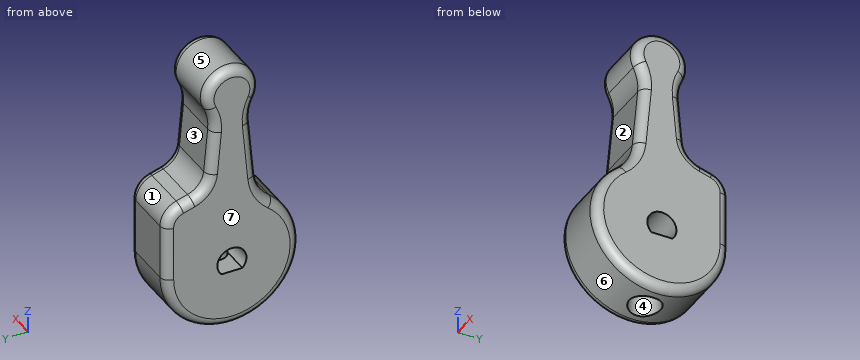
from build123d import *

# Parameters (mm, degrees)
BOSS_EXTRUDE1_DEPTH = 3.5
FILLET1_R           = 5
HOLE1_D             = 2.5
HOLE1_DEPTH         = 8
HOLE1_CBORE_D       = 3.5
HOLE1_CBORE_DEPTH   = 3
BOSS_EXTRUDE2_DEPTH = 7
FILLET3_R           = 2.5
FILLET2_R           = 1


with BuildPart() as part:
    # Sketch1 → Boss-Extrude1 (new, symmetric)
    with BuildSketch(Plane(origin=(0, 0, 0), x_dir=(0, 0, -1), z_dir=(1, 0, 0))):
        with BuildLine():
            Line((-17.763932023, 2), (-6.873863542, 3))
            ThreePointArc((-6.873863542, 3), (7.5, 0), (-6.873863542, -3))
            Line((-6.873863542, -3), (-17.763932023, -2))
            ThreePointArc((-17.763932023, -2), (-23, 0), (-17.763932023, 2))
        make_face()
        with BuildLine():
            Line((1.125, -1.17260394), (1.125, 1.17260394))
            ThreePointArc((1.125, 1.17260394), (-1.625, 0), (1.125, -1.17260394))
        make_face(mode=Mode.SUBTRACT)
    extrude(amount=BOSS_EXTRUDE1_DEPTH, both=True)

    # Fillet1
    fillet1_edges = [part.edges().sort_by_distance(p)[0] for p in [
        (0, 2, 17.763932023),
        (0, 3, 6.873863542),
        (0, -3, 6.873863542),
        (0, -2, 17.763932023),
    ]]
    fillet(fillet1_edges, radius=FILLET1_R)

    # Hole1
    with Locations(Plane(origin=(0, 0, -7.625), x_dir=(1, 0, 0), z_dir=(0, 0, -1))):
        with Locations((0, 0)):
            CounterBoreHole(HOLE1_D / 2, HOLE1_CBORE_D / 2, HOLE1_CBORE_DEPTH, depth=HOLE1_DEPTH)

    # Sketch4 → Boss-Extrude2 (add, through all)
    with BuildSketch(Plane(origin=(3.5, 0, 0), x_dir=(0, 0, -1), z_dir=(1, 0, 0))):
        with BuildLine():
            Line((0, 7.5), (-8, 7.5))
            Line((-8, 7.5), (-9.348908132, 2.772724607))
            ThreePointArc((-9.348908132, 2.772724607), (-7.423390623, 3.356027744), (-5.883671087, 4.651065957))
            ThreePointArc((-5.883671087, 4.651065957), (-3.268562782, 6.750296093), (0, 7.5))
        make_face()
    extrude(amount=-BOSS_EXTRUDE2_DEPTH)

    # Fillet3
    fillet3_edges = [part.edges().sort_by_distance(p)[0] for p in [
        (0, 2.772724607, 9.348908132),
        (0, 7.5, 8),
    ]]
    fillet(fillet3_edges, radius=FILLET3_R)

    # Fillet2
    fillet2_edges = [part.edges().sort_by_distance(p)[0] for p in [
        (-3.5, 0, 23),
        (3.5, 0, 23),
        (-3.5, -3.268562782, -6.750296093),
        (3.5, -3.268562782, -6.750296093),
        (-3.5, -2.469818808, 12.647573032),
        (3.5, -2.469818808, 12.647573032),
        (-3.5, 2.233464618, 17.334759204),
        (3.5, 2.233464618, 17.334759204),
        (-3.5, -3.356027744, 7.423390623),
        (3.5, -3.356027744, 7.423390623),
        (-3.5, -2.233464618, 17.334759204),
        (3.5, -2.233464618, 17.334759204),
        (-3.5, 7.5, 3.056789081),
        (3.5, 7.5, 3.056789081),
        (-3.5, 2.391513819, 13.50031972),
        (3.5, 2.391513819, 13.50031972),
        (3.5, 5.052820312, 8.698292421),
        (-3.5, 5.052820312, 8.698292421),
        (3.5, 6.995615118, 7.619406937),
        (-3.5, 6.995615118, 7.619406937),
        (-3.5, 3.181037085, 9.687418633),
        (3.5, 3.181037085, 9.687418633),
    ]]
    fillet(fillet2_edges, radius=FILLET2_R)


solid = part.part
Design review of the part built by this model. Coordinates are the model's own, in mm. Face numbers are marked on the shaded views. A direction names the side the tool comes from. Give positions to 0.01 mm unless a question says otherwise; leave off trailing zeros. Write each loop counter-clockwise with the first axis right and the second up, starting at its lowest first coordinate (ties: lowest second). Pieces come first, ordered by that corner, then holes. Notation, with made-up numbers: M 36,6.25 L 74,6.25 A25 ccw 74,35.25 Z; hole C 33,-31.75 d2. An arc over 180 degrees is marked long. Answer as a JSON object with one key per item and string values. Group by question number.
1) We need section C-C (x = 0). Give the boundary of the cut face in (y, z) (3 decimals), and give its area (3 significant figures).
2) For line 1 along Y through (x, z) = (-0.5, -2); line 2 along Y through (x, z) = (0, -5.4); line 3 along Z through (x, y) = (2.75, 0.25) (3 decimals), list the stretches that pass through material, from the lowest coordinate up.
3) Mouldability with a two-part tool opening along Z and no side actions: class the marked faces 5, 6 and 7 as released by +Z, released by -Z, zero draft, split by the parting line, or undercut.
4) We need section A-A (y = 0). Give the boundary of the cut face in (x, z) (3 decimals), and give its area (3 significant figures).
5) Tool access review of the marked faces 1, 2, 3 and 4: name each direction out of +Z, -Z, +X, -X, +Y, -Y from which nothing blocks a thin tool from reaching the whole face with its end or side.
6) Clearance check with flat-ended pins moving along their axes: pin 1 Ø2 at (x, z) = (2.5, 11.5) entering from -Y; pin 2 Ø2 at (x, y) = (0, 0) entering from -Z. State where each tip first meets the part, or that it passes through.
Answer key:
{
 "1": {"outline": "M -4.651,5.884 A7.5 ccw -1.75,-7.293 L -1.75,-4.625 L -1.25,-4.625 L -1.25,-1.038 A1.625 cw long 1.25,-1.038 L 1.25,-4.625 L 1.75,-4.625 L 1.75,-7.293 A7.5 ccw 7.5,0 L 7.5,6.114 A2.5 ccw 5.686,8.518 L 4.42,8.879 A2.5 cw 2.616,11.054 L 2.167,15.946 A5 cw 2.68,18.651 A3 ccw long -2.68,18.651 A5 cw -2.167,15.946 L -2.773,9.349 A5 cw Z", "area": "247 mm²"},
 "2": {"line 1": "y = -7.23 to -1.15, 1.15 to 7.23", "line 2": "y = -5.2 to -1.75, 1.75 to 5.2", "line 3": "z = -7.464 to -1.125, 1.606 to 22.958"},
 "3": {"face 5": "undercut", "face 6": "split by the parting line", "face 7": "zero draft"},
 "4": {"outline": "M -3.5,-6.5 A1 ccw -2.5,-7.5 L -1.75,-7.5 L -1.75,-4.625 L -1.25,-4.625 L -1.25,-1.125 L -3.5,-1.125 Z; M -3.5,1.625 L 3.5,1.625 L 3.5,22 A1 ccw 2.5,23 L -2.5,23 A1 ccw -3.5,22 Z; M 1.25,-4.625 L 1.75,-4.625 L 1.75,-7.5 L 2.5,-7.5 A1 ccw 3.5,-6.5 L 3.5,-1.125 L 1.25,-1.125 Z", "area": "175 mm²"},
 "5": {"face 1": "+Z, +X, -X, +Y", "face 2": "+X, -X, -Y", "face 3": "+X, -X, +Y", "face 4": "-Z"},
 "6": {"pin 1": "stops at y = -2.67", "pin 2": "stops at z = 1.28"}
}
